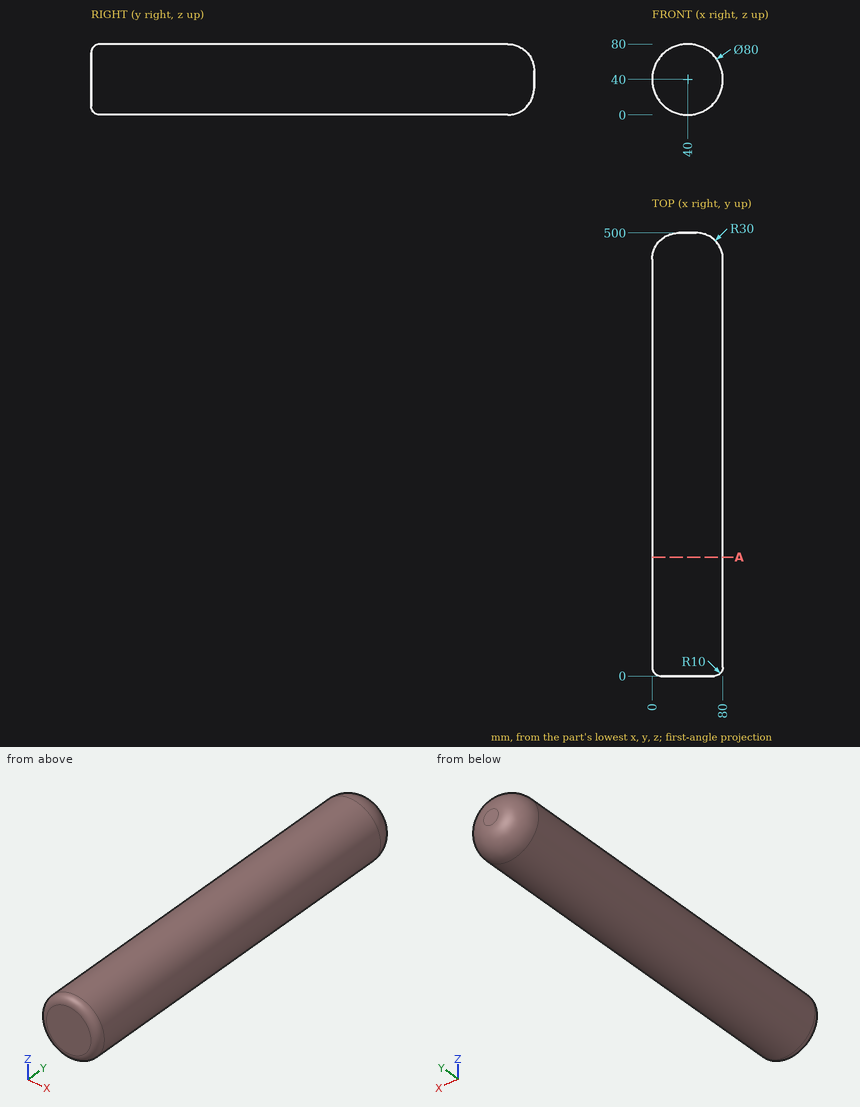
Verification items for this drawing (mm, ordinates from the low corner). Round coordinates to 2 decimals unless told otherwise and drop trailing zeros. Order: outer loops, then holes, each group sorted by start corner. A loop starts at its lowest first (then second) coordinate and runs counter-clockwise, first axis right, second up. Notation, with made-up numbers: (79, 36.25) - (131, 36.25) arc R19 cw to (131, 54.25) - close; hole circle Ø11 at (50, -22.75). An arc over 180 degrees is marked (long way). Use CSV: the item, a comma, the result in double quotes. Start each with the question number.
1) Thickness scan on L1, parallel to Y at x = 28, z = 40; L2, parallel to X at y = 316.5, z = 41.5; L3, parallel to Z at x = 28.5, y = 74.5. Record the ranges inside material, lowest first.
2) Section check A-A, the plane y = 134. Record the cut outline in (x, z).
3) Go/stop test with flat-tipped pins: P1, Ø1, axis at x = 65.5, z = 69, coming from the -Y side; P2, Ø6, axis at y = 137.5, z = 63, coming from the +X side; P3, Ø4, axis at y = 161.5, z = 18.5, coming from the +X side. Record where each tip stops, or that it passes through.
Answers:
1,L1,"y = 0 to 499.93"
1,L2,"x = 0.03 to 79.97"
1,L3,"z = 1.69 to 78.31"
2,outline,"circle Ø80 at (40, 40)"
3,P1,"stops at y = 4.16"
3,P2,"stops at x = 74.64"
3,P3,"stops at x = 74.92"
